Can you work these out from the model? Positions are in its coordinate system, mm. Face numbers are marked on the shaded views. Round coordinates to 2 decimals unless told otherwise and drop trailing zeros. Write each loop counter-clockwise with the first axis right and the second up, starting at its lowest first coordinate (ties: lowest second). Pieces come first, ordered by that corner, then holes. Notation, with made-up numbers: (42, 84.25) - (79, 84.25) arc R18 cw to (79, 108.25) - close; hole circle Ø10 at (-11, 87.25). An arc over 180 degrees is marked (long way). One line per item, written item: value. Start each with the question number.
(1) If I drill on L1, parallel to Z at x = -50, y = 5; L2, parallel to X at y = 4, z = 0; L3, parallel to X at y = 9.5, z = 0, over which ranges is the centre line in solid material (lowest first)? Write a range as from..to.
(2) Thinking about a two-plate mould opening in X: for the marked faces 1 and 2, which applies, +X half, -X half, draft (parallel to the pull), parting line (faces both ways), or undercut?
(3) I want a section at B-B on x = -29. List the corners of the cut face in (y, z) for me, plus the area to 3 significant figures.
(4) I want a section at C-C on z = 28. List the corners of the cut face in (x, y) for me, plus the area to 3 significant figures.
(5) I'm going to push flat-ended pins straight in: pin 1 Ø11 at (x, z) = (-1.5, -2) entering from +Y; pin 2 Ø3.5 at (x, y) = (-3.5, 13) entering from +Z; pin 3 Ø4 at (x, z) = (58.5, 0) entering from +Y. Where does each tip first touch, or does it pass through?
from build123d import *

# Parameters (mm, degrees)
SKETCH1_W           = 130
SKETCH1_H           = 60
SKETCH1_R           = 2.15
SKETCH1_R_2         = 2.65
BOSS_EXTRUDE1_DEPTH = 14
CUT_EXTRUDE1_DEPTH  = 7
SKETCH3_R           = 4.1
CUT_EXTRUDE2_DEPTH  = 7
SKETCH4_W           = 96
SKETCH4_H           = 36
CUT_EXTRUDE3_DEPTH  = 3
CUT_EXTRUDE4_DEPTH  = 130
FILLET1_R           = 1.5


with BuildPart() as part:
    # Sketch1 → Boss-Extrude1 (new body)
    with BuildSketch(Plane(origin=(0, 0, 0), x_dir=(1, 0, 0), z_dir=(0, 1, 0))):
        Rectangle(SKETCH1_W, SKETCH1_H)
        with Locations((-43.5, 4.3)):
            Circle(SKETCH1_R, mode=Mode.SUBTRACT)
        with Locations((43.5, 4.3)):
            Circle(SKETCH1_R, mode=Mode.SUBTRACT)
        with Locations((-57, 0)):
            Circle(SKETCH1_R_2, mode=Mode.SUBTRACT)
        with Locations((57, 0)):
            Circle(SKETCH1_R_2, mode=Mode.SUBTRACT)
    extrude(amount=BOSS_EXTRUDE1_DEPTH)

    # Sketch2 → Cut-Extrude1 (cut)
    with BuildSketch(Plane.XZ):
        Polygon((-39.577622793, -5.676574387), (-40.346663007, -1.591408889), (-44.269040214, -0.214834502), (-47.422377207, -2.923425613), (-46.653336993, -7.008591111), (-42.730959786, -8.385165498), align=None)
        Polygon((42.815034421, -8.400100262), (46.708308195, -6.943247723), (47.393273774, -2.843147461), (44.184965579, -0.199899738), (40.291691805, -1.656752277), (39.606726226, -5.756852539), align=None)
    extrude(amount=-CUT_EXTRUDE1_DEPTH, mode=Mode.SUBTRACT)

    # Sketch3 → Cut-Extrude2 (cut)
    with BuildSketch(Plane(origin=(0, 14, 0), x_dir=(1, 0, 0), z_dir=(0, 1, 0))):
        with Locations((-57, 0)):
            Circle(SKETCH3_R)
        with Locations((57, 0)):
            Circle(SKETCH3_R)
    extrude(amount=-CUT_EXTRUDE2_DEPTH, mode=Mode.SUBTRACT)

    # Sketch4 → Cut-Extrude3 (cut)
    with BuildSketch(Plane(origin=(0, 14, 0), x_dir=(1, 0, 0), z_dir=(0, 1, 0))):
        Rectangle(SKETCH4_W, SKETCH4_H)
    extrude(amount=-CUT_EXTRUDE3_DEPTH, mode=Mode.SUBTRACT)

    # Sketch5 → Cut-Extrude4 (cut)
    with BuildSketch(Plane(origin=(65, 0, 0), x_dir=(0, 0, -1), z_dir=(1, 0, 0))):
        with BuildLine():
            Line((-24, 14), (-24, 8.5))
            Line((-24, 8.5), (-26.5, 8.5))
            Line((-26.5, 8.5), (-26.5, 10))
            ThreePointArc((-26.5, 10), (-28, 11.5), (-29.5, 10))
            Line((-29.5, 10), (-29.5, 4))
            ThreePointArc((-29.5, 4), (-28, 2.5), (-26.5, 4))
            Line((-26.5, 4), (-26.5, 5.5))
            Line((-26.5, 5.5), (-24, 5.5))
            Line((-24, 5.5), (-24, 0))
            Line((-24, 0), (-30, 0))
            Line((-30, 0), (-30, 14))
            Line((-30, 14), (-24, 14))
        make_face()
        with BuildLine():
            Line((27.85, 8.8), (30, 8.8))
            Line((30, 8.8), (30, 5.2))
            Line((30, 5.2), (27.85, 5.2))
            Line((27.85, 5.2), (27.85, 3.85))
            ThreePointArc((27.85, 3.85), (26.2, 2.2), (24.55, 3.85))
            Line((24.55, 3.85), (24.55, 10.15))
            ThreePointArc((24.55, 10.15), (26.2, 11.8), (27.85, 10.15))
            Line((27.85, 10.15), (27.85, 8.8))
        make_face()
    extrude(amount=-CUT_EXTRUDE4_DEPTH, mode=Mode.SUBTRACT)

    # Fillet1
    fillet1_edges = [part.edges().sort_by_distance(p)[0] for p in [
        (65, 0, -3),
        (65, 14, -3),
        (0, 14, 24),
        (0, 0, 24),
        (-65, 14, -3),
        (-65, 0, -3),
        (0, 0, -30),
        (0, 14, -30),
    ]]
    fillet(fillet1_edges, radius=FILLET1_R)


solid = part.part
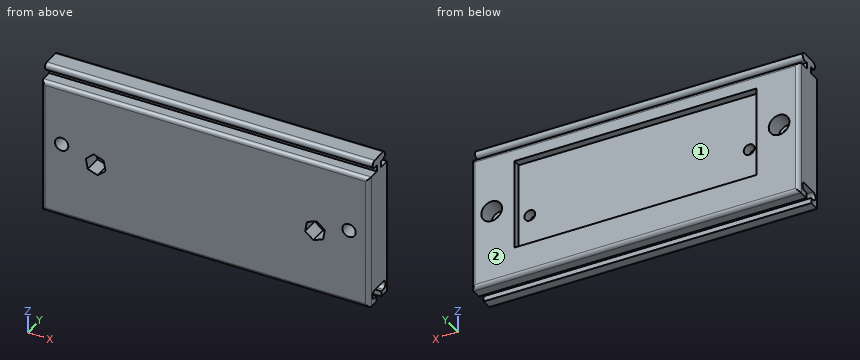
Established:
1. L1: -30..-27.85, -24.55..24, 26.5..29.5
1. L2: -65..-59.65, -54.35..54.35, 59.65..65
1. L3: -65..-61.1, -52.9..52.9, 61.1..65
2. face 1: undercut
2. face 2: draft
3. outline: (0, -28.5) arc R1.5 ccw to (1.5, -30) - (5.2, -30) - (5.2, -27.85) - (3.85, -27.85) arc R1.65 cw to (3.85, -24.55) - (10.15, -24.55) arc R1.65 cw to (10.15, -27.85) - (8.8, -27.85) - (8.8, -30) - (12.5, -30) arc R1.5 ccw to (14, -28.5) - (14, -18) - (11, -18) - (11, 18) - (14, 18) - (14, 22.5) arc R1.5 ccw to (12.5, 24) - (8.5, 24) - (8.5, 26.5) - (10, 26.5) arc R1.5 ccw to (10, 29.5) - (4, 29.5) arc R1.5 ccw to (4, 26.5) - (5.5, 26.5) - (5.5, 24) - (1.5, 24) arc R1.5 ccw to (0, 22.5) - close
3. area: 642 mm2
4. outline: (-65, 2.5) - (65, 2.5) - (65, 11.5) - (-65, 11.5) - close
4. area: 1,170 mm2
5. pin 1: y = 11
5. pin 2: z = 28.83
5. pin 3: y = 7
